Could you check a few things on this drawing? It's one solid part, dimensions in mm from its lowest x, y, z. A direction names the side the tool comes from. Coordinates: 2 decimals unless noted, no trailing zeros. Order: outer loops, then holes, each group sorted by start corner. A loop starts at its lowest first (then second) coordinate and runs counter-clockwise, first axis right, second up. Notation, with made-up numbers: (-40, 71) -> (5, 71) arc R22 ccw to (5, 82) -> close; hole circle Ø5 at (47.25, -10.75). An arc over 180 degrees is marked (long way). Use a Markdown table: item, result. Add a question column.
1. Suppose I cut it at D-D, the plane y = 23.5. List the corners of the cut face in (x, z) for me, then the cut area to 3 significant figures.
2. For pin 1 Ø15.5 at (x, y) = (11.5, 18.5) entering from +Z; pin 2 Ø0.9 at (x, z) = (5.5, 7.5) entering from -Y; pin 3 Ø0.9 at (x, z) = (8, 8) entering from +Y, each with a flat end and sliding along its axis, tell me the tip position at first contact or that it passes through.
3. Suppose I cut it at C-C, the plane z = 11. List the corners of the cut face in (x, y) for me, then the cut area to 3 significant figures.
4. If I drill on line 1 along Y through (x, z) = (40, 5); line 2 along X through (y, z) = (30, 1); line 3 along Z through (x, y) = (15, 22), over which ranges is the centre line in solid material (lowest first)? Write a range as from..to.
5. Suppose I cut it at B-B, the plane x = 40. List the corners of the cut face in (y, z) for me, then the cut area to 4 significant figures.
6. We'd pull the mould along Y, two halves only. Please class the marked faces 3, 4, 5 and 6: pulls with the +Y half, pulls with the -Y half, needs draft (parallel to the pull), parting line crosses it, or undercut.
7. For the marked faces 1 and 2, which set-ups out of +Z, -Z, +X, -X, +Y, -Y let a thin tool reach every point of the face, with its end or its side?
8. Suppose I cut it at A-A, the plane y = 15.75. List the corners of the cut face in (x, z) for me, then the cut area to 3 significant figures.
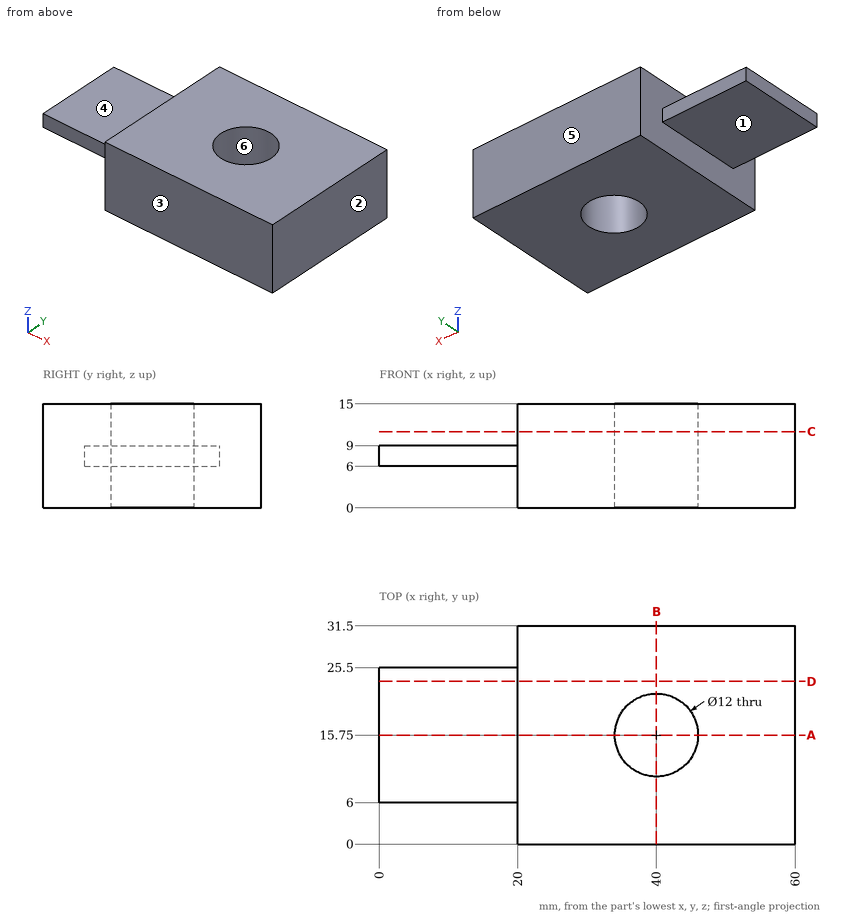
Worked out:
| question | item | result |
|---|---|---|
| 1 | outline | (0, 6) -> (20, 6) -> (20, 0) -> (60, 0) -> (60, 15) -> (20, 15) -> (20, 9) -> (0, 9) -> close |
| 1 | area | 660 mm² |
| 2 | pin 1 | stops at z = 9 |
| 2 | pin 2 | stops at y = 6 |
| 2 | pin 3 | stops at y = 25.5 |
| 3 | outline | (20, 0) -> (60, 0) -> (60, 31.5) -> (20, 31.5) -> close; hole circle Ø12 at (40, 15.75) |
| 3 | area | 1,150 mm² |
| 4 | line 1 | y = 0..9.75, 21.75..31.5 |
| 4 | line 2 | x = 20..60 |
| 4 | line 3 | z = 6..9 |
| 5 | outline | (0, 0) -> (9.75, 0) -> (9.75, 15) -> (0, 15) -> close; (21.75, 0) -> (31.5, 0) -> (31.5, 15) -> (21.75, 15) -> close |
| 5 | area | 292.5 mm² |
| 6 | face 3 | pulls with the -Y half |
| 6 | face 4 | needs draft |
| 6 | face 5 | pulls with the +Y half |
| 6 | face 6 | undercut |
| 7 | face 1 | -Z, -X, +Y, -Y |
| 7 | face 2 | +Z, -Z, +X, +Y, -Y |
| 8 | outline | (0, 6) -> (20, 6) -> (20, 0) -> (34, 0) -> (34, 15) -> (20, 15) -> (20, 9) -> (0, 9) -> close; (46, 0) -> (60, 0) -> (60, 15) -> (46, 15) -> close |
| 8 | area | 480 mm² |
